Work out the finished part from the listing and answer in its coordinate system (mm). Face numbers are marked on the shaded views. A direction names the side the tool comes from. Round coordinates to 2 decimals unless told otherwise and drop trailing zeros. Loops run counter-clockwise (first coordinate to the right, second up) from the corner with the lowest first, then second, coordinate; pieces in that order, holes last. Notation, with made-up numbers: (-18, 78.5) - (40, 78.5) arc R10 ccw to (40, 86.5) - close; hole circle Ø1 at (16.5, -28.75). An arc over 180 degrees is marked (long way). Return JSON: item names as keys, results as strings.
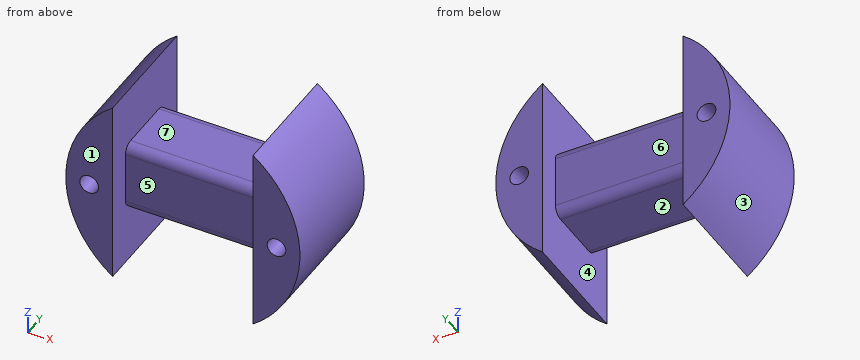
from build123d import *

# Parameters (mm, degrees)
F0_R          = 2
F1_DEPTH      = 25
F2_W          = 30
F2_H          = 12.4809114001
F3_DEPTH      = 25
F3_DEPTH_BACK = 25
F4_R          = 2


with BuildPart() as f1:
    # F0 (on Front) → F1 (new body)
    with BuildSketch(Plane.XZ):
        with BuildLine():
            Line((-15, 7.5), (-15, 20))
            ThreePointArc((-15, 20), (-25, 0), (-15, -20))
            Line((-15, -20), (-15, -7.5))
            Line((-15, -7.5), (15, -7.5))
            Line((15, -7.5), (15, -20))
            ThreePointArc((15, -20), (25, 0), (15, 20))
            Line((15, 20), (15, 7.5))
            Line((15, 7.5), (-15, 7.5))
        make_face()
        with Locations((-20, 0)):
            Circle(F0_R, mode=Mode.SUBTRACT)
        with Locations((20, 0)):
            Circle(F0_R, mode=Mode.SUBTRACT)
    extrude(amount=F1_DEPTH)

    # F2 (on Top) → F3 (cut, two sides)
    with BuildSketch(Plane.XY) as f3_sk:
        with Locations((0, 1.2404557001)):
            Rectangle(F2_W, F2_H)
        with Locations((0, -26.2404557001)):
            Rectangle(F2_W, F2_H)
    extrude(amount=-F3_DEPTH, mode=Mode.SUBTRACT)
    extrude(f3_sk.sketch, amount=F3_DEPTH_BACK, mode=Mode.SUBTRACT)

    # F4
    f4_edges = [f1.edges().sort_by_distance(p)[0] for p in [
        (0, -20, 7.5),
        (0, -20, -7.5),
        (0, -5, -7.5),
        (0, -5, 7.5),
    ]]
    fillet(f4_edges, radius=F4_R)


solid = f1.part
1) Find the intervals of material crossed by L1, parallel to Z at x = 20, y = -15.25; L2, parallel to Z at x = 5.5, y = -10.75; L3, parallel to Y at x = -7, z = 1.5, in increasing order.
Verdict:
{"L1": "z = -15 to -2, 2 to 15", "L2": "z = -7.5 to 7.5", "L3": "y = -20 to -5"}
2) Determine the mould class of the marked faces 1, 2, 3 and 4 for opening direction X: pulls with the +X half, pulls with the -X half, needs draft (parallel to the pull), parting line crosses it, or undercut.
Verdict:
{"face 1": "needs draft", "face 2": "undercut", "face 3": "pulls with the -X half", "face 4": "undercut"}
3) Section C-C (y = -17.25) is taken. Give the vertices of the cut face in (x, z).
Verdict:
{"outline": "(-15, -20) - (-15, -7.5) - (15, -7.5) - (15, -20) arc R25 ccw to (15, 20) - (15, 7.5) - (-15, 7.5) - (-15, 20) arc R25 ccw to start; hole circle Ø4 at (-20, 0); hole circle Ø4 at (20, 0)"}
4) Section B-B (z = 9.5) is taken. Give the vertices of the cut face in (x, y).
Verdict:
{"outline": "(-23.12, -25) - (-15, -25) - (-15, 0) - (-23.12, 0) - close; (15, -25) - (23.12, -25) - (23.12, 0) - (15, 0) - close"}
5) Section A-A (x = 20) is taken. Give the vertices of the cut face in (y, z).
Verdict:
{"outline": "(-25, -15) - (0, -15) - (0, -2) - (-25, -2) - close; (-25, 2) - (0, 2) - (0, 15) - (-25, 15) - close"}
6) Flat-ended cylindrical pins translate along their axes: pin 1 (4 mm diameter, centred on x = -7.5, y = -21.5, fed in from +Z); pin 2 (9 mm diameter, centred on x = -2, z = 0.5, fed in from +Y); pin 3 (3 mm diameter, centred on y = -17.5, z = 14.5, fed in from -X). Find the tip coordinate at first contact, or state that the pin passes through.
Verdict:
{"pin 1": "stops at z = 6.82", "pin 2": "stops at y = -5", "pin 3": "stops at x = -21.35"}
7) Section D-D (z = 1) is taken. Give the vertices of the cut face in (x, y), and give its area (3 significant figures).
Verdict:
{"outline": "(-24.98, -25) - (-21.73, -25) - (-21.73, 0) - (-24.98, 0) - close; (-18.27, -25) - (-15, -25) - (-15, -20) - (15, -20) - (15, -25) - (18.27, -25) - (18.27, 0) - (15, 0) - (15, -5) - (-15, -5) - (-15, 0) - (-18.27, 0) - close; (21.73, -25) - (24.98, -25) - (24.98, 0) - (21.73, 0) - close", "area": "776 mm2"}
8) A tool of negligible diameter and unlimited length cuts with its end or side. For the marked faces 5, 6 and 7, from which of +Z, -Z, +X, -X, +Y, -Y can it reach the whole face along a straight path? Write none if from no direction.
Verdict:
{"face 5": "+Z, -Z, -Y", "face 6": "+Z, -Z, +Y", "face 7": "+Z, +Y, -Y"}
